Autodesk Inventor part; units mm, degrees
ref_plane "YZ Plane" through (0, 0, 0) normal (1, 0, 0) x (0, 1, 0)
ref_plane "XZ Plane" through (0, 0, 0) normal (0, 1, 0) x (-1, 0, 0)
ref_plane "XY Plane" through (0, 0, 0) normal (0, 0, 1) x (1, 0, 0)
sketch "スケッチ1" plane through (0, 0, 0) normal (0, 0, 1) x (1, 0, 0)
  line L0 (-24.25, -20) -> (24.25, -20) construction
  line L1 (24.25, -20) -> (24.25, 20)
  line L2 (24.25, 20) -> (-24.25, 20)
  line L3 (-24.25, 20) -> (-24.25, -20)
  line L4 (-24.25, -20) -> (24.25, 20) construction
  line L5 (24.25, -20) -> (-24.25, 20) construction
  circle A0 centre (-15.25, -17.5) radius 1.55
  circle A1 centre (20.25, -17.5) radius 1.55
  line L6 (-9.25, -15) -> (14.25, -15) construction
  line L7 (14.25, -15) -> (14.25, -20) construction
  line L8 (14.25, -20) -> (-9.25, -20) construction
  line L9 (-9.25, -20) -> (-9.25, -15) construction
  line L10 (-24.25, -20) -> (-15.25, -22)
  line L11 (-15.25, -22) -> (20.25, -22)
  line L12 (20.25, -22) -> (24.25, -20)
  line L13 (14.3, -14.95) -> (-9.3, -14.95)
  line L14 (-9.3, -14.95) -> (-9.3, -20.05)
  line L15 (-9.3, -20.05) -> (14.3, -20.05)
  line L16 (14.3, -20.05) -> (14.3, -14.95)
  circle A2 centre (-8.25, -14.95) radius 1.05
  circle A3 centre (-8.25, -20.05) radius 1.05
  circle A4 centre (13.25, -14.95) radius 1.05
  circle A5 centre (13.25, -20.05) radius 1.05
  circle A6 centre (-19.25, 15) radius 1.55
  line L17 (-21.8, 5.05) -> (-19.2, 5.05)
  line L18 (-19.2, 5.05) -> (-19.2, -15.05)
  line L19 (-19.2, -15.05) -> (-21.8, -15.05)
  line L20 (-21.8, -15.05) -> (-21.8, 5.05)
  line L21 (-19.25, 5) -> (-21.75, 5) construction
  line L22 (-21.75, 5) -> (-21.75, -15) construction
  line L23 (-21.75, -15) -> (-19.25, -15) construction
  line L24 (-19.25, -15) -> (-19.25, 5) construction
  line L25 (2.5, -14.95) -> (2.5, -20.05) construction
  circle A7 centre (-21.8, 4) radius 1.05
  circle A8 centre (-19.2, 4) radius 1.05
  circle A9 centre (-21.8, -14) radius 1.05
  circle A10 centre (-19.2, -14) radius 1.05
  point P0 (0, 0)
  point P1 (0, 0)
  point P2 (-9.25, -17.5)
  dimension "d8" = 2.1
  dimension "d22" = 2.1
  dimension "d1" = 5
  dimension "d2" = 3.1
  dimension "d3" = 35.5
  dimension "d4" = 2
  dimension "d5" = 40
  dimension "d6" = 23.5
  dimension "d7" = 0.05
  dimension "d9" = 3.1
  dimension "d10" = 5
  dimension "d11" = 5
  dimension "d12" = 0.05
  dimension "d13" = 17.75
  dimension "d14" = 48.5
  dimension "d15" = 4
  dimension "d18" = 2.5
  dimension "d19" = 2.5
  dimension "d20" = 5
  dimension "d21" = 15
  dimension "d23" = 25
extrude "押し出し1" add sketch "スケッチ1" along normal blind 5
sketch "スケッチ3" plane through (0, 0, 5) normal (0, 0, 1) x (1, 0, 0)
  line L0 (-15.2, 16) -> (20.25, 16)
  line L1 (20.25, 16) -> (20.25, -10.95)
  line L2 (20.25, -10.95) -> (-15.2, -10.95)
  line L3 (-15.2, -10.95) -> (-15.2, 16)
  line L4 (24.25, -20) -> (24.25, 20)
  line L5 (24.25, 20) -> (-24.25, 20)
  line L6 (-7.2, -14.95) -> (12.2, -14.95)
  line L7 (-19.2, 2.95) -> (-19.2, -12.95)
  point P0 (0, 0)
  dimension "d26" = 4
  dimension "d27" = 4
  dimension "d28" = 4
  dimension "d29" = 4
extrude "押し出し2" cut sketch "スケッチ3" against normal blind 3
sketch "スケッチ4" plane through (0, 0, 5) normal (0, 0, 1) x (1, 0, 0)
  circle A0 centre (-15.25, -17.5) radius 3
  circle A1 centre (20.25, -17.5) radius 3
  circle A2 centre (-15.25, -17.5) radius 1.55
  circle A3 centre (20.25, -17.5) radius 1.55
  point P0 (0, 0)
  dimension "d32" = 6
  dimension "d33" = 6
extrude "押し出し3" cut sketch "スケッチ4" against normal blind 3.5
fillet "フィレット1" radius 2 4 edges at (-15.2, 16, 3.5) (-15.2, -10.95, 3.5) (20.25, -10.95, 3.5) (20.25, 16, 3.5)
sketch "スケッチ10" plane through (24.25, -20, 0) normal (1, 0, 0) x (0, 0, -1)
  line L0 (-5, 40) -> (-5, 0)
  line L1 (-5, 33) -> (0, 33)
  line L2 (0, 33) -> (0, 18)
  line L3 (0, 18) -> (-5, 18)
  line L4 (-5, 18) -> (-5, 33)
  line L5 (0, 40) -> (-5, 40)
  point P0 (0, 20)
  dimension "d52" = 5
  dimension "d53" = 15
  dimension "d54" = 7
extrude "押し出し9" add sketch "スケッチ10" along normal blind 1.75
sketch "スケッチ11" plane through (0, 0, 0) normal (0, 0, -1) x (-1, 0, 0)
  line L0 (-24.25, -2) -> (-26, -2)
  line L1 (-26, -2) -> (-26, 13)
  line L2 (-24.25, 13) -> (-24.25, 20)
  line L3 (-26, 13) -> (-24.25, 13)
  line L4 (-26, -2) -> (-26, 13)
  line L5 (-24.25, 13) -> (-26, -2)
  point P0 (0, 0)
extrude "押し出し10" cut sketch "スケッチ11" against normal through all
fillet "フィレット2" radius 0.8 1 edges at (26, -2, 2.5)
fillet "フィレット3" radius 0.5 1 edges at (24.25, -2, 2.5)
equation "\"d11\" = d10"
equation "\"d13\" = 0.5 * d3"
equation "\"d27\" = d26"
equation "\"d28\" = d26"
equation "\"d29\" = d26"
properties part number "コックピット_サブフレーム_1_5_MIR" material "アセタール樹脂、黒"
The listing builds one solid part. Answer for the finished solid, in the listing's coordinates (mm). A direction names the side the tool comes from. Round coordinates to 2 decimals unless told otherwise and drop trailing zeros. Loops run counter-clockwise (first coordinate to the right, second up) from the corner with the lowest first, then second, coordinate; pieces in that order, holes last. Notation, with made-up numbers: (-23.5, 26.25) - (17.5, 26.25) arc R10 cw to (17.5, 34.25) - close; hole circle Ø6 at (-23.75, -34.5). An arc over 180 degrees is marked (long way). Return JSON: item names as keys, results as strings. Group by question number.
1. The mould has two halves that part along X. Classify faces 4 (the flat face through (25.06, 6.05, 2.46)), 5 (the cylindrical face through (-22.85, 3.98, 2.46)), 6 (the flat face through (-24.25, 0, 2)): pulls with the +X half, pulls with the -X half, needs draft (parallel to the pull), parting line crosses it, or undercut.
2. Each of these flat-tipped pins is pushed along its axis until it touches: P1, Ø3.5, axis at x = 20.25, y = -17.5, coming from the +Z side; P2, Ø2, axis at y = 0.5, z = 2, coming from the +X side (3 decimals); P3, Ø1.5, axis at y = 8, z = 3.5, coming from the +X side. Where does it stop, or does it pass through?
3. The part is cut by section A-A on x = -8.25. Determine the outline of the cut face in (y, z).
4. Consider probe 1 along Y at (x, z) = (-19.25, 2.7); probe 2 along X at (y, z) = (-1, 4.75); probe 3 along Y at (x, z) = (3, 2.8). Determine where each line is inside the solid, lowest interval first.
5. The part is cut by section C-C on y = 4. Determine the outline of the cut face in (x, z), then the cut area to 3 significant figures.
6. The part is cut by section B-B on y = -17.5. Determine the outline of the cut face in (x, z), then the cut area to 3 significant figures.
7. The part is cut by section D-D on z = 4.4. State how many separate pieces and enclosed holes the cut face has, then the cut area to 3 significant figures.
8. Which of the six approach directions +Z, -Z, +X, -X, +Y, -Y give full straight-line access (tool end or side, diameter ignored) to faces 1 (the cylindrical face through (19.65, 15.43, 3.48)), 2 (the flat face through (-19.813, -20.986, 2.465)), 3 (the cylindrical face through (13.3, -21.1, 2.5))?
Resolved:
{
 "1": {"face 4": "pulls with the +X half", "face 5": "undercut", "face 6": "pulls with the -X half"},
 "2": {"P1": "stops at z = 1.5", "P2": "stops at x = 25.825", "P3": "stops at x = 24.92"},
 "3": {"outline": "(-22, 0) - (-21.1, 0) - (-21.1, 5) - (-22, 5) - close; (-13.9, 0) - (20, 0) - (20, 5) - (16, 5) - (16, 2) - (-10.95, 2) - (-10.95, 5) - (-13.9, 5) - close"},
 "4": {"probe 1": "y = -21.11 to -15.05, 5.05 to 13.45, 16.55 to 20", "probe 2": "x = -24.25 to -21.8, -19.2 to -15.2, 20.25 to 25.88", "probe 3": "y = -22 to -20.05, -14.95 to -10.95, 16 to 20"},
 "5": {"outline": "(-24.25, 0) - (-22.85, 0) - (-22.85, 5) - (-24.25, 5) - close; (-18.15, 0) - (25.3, 0) - (25.3, 5) - (20.25, 5) - (20.25, 2) - (-15.2, 2) - (-15.2, 5) - (-18.15, 5) - close", "area": "118 mm²"},
 "6": {"outline": "(-24.25, 0) - (-16.8, 0) - (-16.8, 1.5) - (-18.25, 1.5) - (-18.25, 5) - (-24.25, 5) - close; (-13.7, 0) - (-9.3, 0) - (-9.3, 5) - (-12.25, 5) - (-12.25, 1.5) - (-13.7, 1.5) - close; (14.3, 0) - (18.7, 0) - (18.7, 1.5) - (17.25, 1.5) - (17.25, 5) - (14.3, 5) - close; (21.8, 0) - (24.25, 0) - (24.25, 5) - (23.25, 5) - (23.25, 1.5) - (21.8, 1.5) - close", "area": "73.2 mm²"},
 "7": {"separate pieces": "1", "enclosed holes": "6", "area": "834 mm²"},
 "8": {"face 1": "+Z", "face 2": "+Z, -Z, -X, -Y", "face 3": "+Z, -Z"}
}
